```python
from build123d import *

# Parameters (mm, degrees)
SKETCH1_R           = 15
BOSS_EXTRUDE1_DEPTH = 5
SKETCH2_R           = 10
BOSS_EXTRUDE2_DEPTH = 15
SKETCH3_R           = 7.5
CUT_EXTRUDE1_DEPTH  = 19
SKETCH5_R           = 11
BOSS_EXTRUDE3_DEPTH = 1


with BuildPart() as part:
    # Sketch1 → Boss-Extrude1 (new body)
    with BuildSketch(Plane(origin=(0, 0, 0), x_dir=(1, 0, 0), z_dir=(0, 1, 0))):
        Circle(SKETCH1_R)
    extrude(amount=BOSS_EXTRUDE1_DEPTH)

    # Sketch2 → Boss-Extrude2 (add)
    with BuildSketch(Plane(origin=(0, 5, 0), x_dir=(1, 0, 0), z_dir=(0, 1, 0))):
        Circle(SKETCH2_R)
    extrude(amount=BOSS_EXTRUDE2_DEPTH)

    # Sketch3 → Cut-Extrude1 (cut)
    with BuildSketch(Plane.XZ):
        Circle(SKETCH3_R)
    extrude(amount=-CUT_EXTRUDE1_DEPTH, mode=Mode.SUBTRACT)

    # Sketch5 → Boss-Extrude3 (add)
    with BuildSketch(Plane(origin=(0, 5, 0), x_dir=(1, 0, 0), z_dir=(0, 1, 0))):
        Circle(SKETCH5_R)
    extrude(amount=BOSS_EXTRUDE3_DEPTH)


solid = part.part
```
The listing builds one solid part. Answer for the finished solid, in the listing's coordinates (mm). A direction names the side the tool comes from. Give positions to 0.01 mm unless a question says otherwise; leave off trailing zeros. Loops run counter-clockwise (first coordinate to the right, second up) from the corner with the lowest first, then second, coordinate; pieces in that order, holes last. Notation, with made-up numbers: (-12.75, 78) - (5.25, 78) arc R22 ccw to (5.25, 94) - close; hole circle Ø5 at (-10, 63.5). An arc over 180 degrees is marked (long way). Return JSON: item names as keys, results as strings. Group by question number.
1. Straight lines are drawn through the part: line 1 (Y direction, x = 2.5, z = 1.5); line 2 (Z direction, x = 0, y = 12.75); line 3 (Z direction, x = 0, y = 1.8). For each, find the intervals that lie inside material, in ascending order. Write a range as [from, to].
2. Find section A-A (x = 0). Write down the section's boundary in (y, z).
3. Determine the mould class of faces 1 (the cylindrical face through (-14.985, 2.465, -0.66)), 2 (the cylindrical face through (-7.493, 2.465, 0.33)), 3 (the flat face through (0, 6, 0)), 4 (the flat face through (2, 6, 10)) for opening direction Z: pulls with the +Z half, pulls with the -Z half, needs draft (parallel to the pull), parting line crosses it, or undercut.
4. Which of the six approach directions +Z, -Z, +X, -X, +Y, -Y give full straight-line access (tool end or side, diameter ignored) to faces 5 (the flat face through (0, 20, 0)), 6 (the flat face through (0, 5, 0)), 7 (the cylindrical face through (-7.493, 12.409, 0.33)), 8 (the cylindrical face through (-2.17, 12.9, 9.76)), 9 (the flat face through (-4, 0, -7))?
5. Find section D-D (z = -8.25). Write down the section's boundary in (x, y).
6. Find section C-C (y = 4). Write down the section's boundary in (x, z), then the cut area to 3 significant figures.
7. Given pin 1 Ø8 at (y, z) = (16, 0.5) entering from +X; pin 2 Ø1.5 at (x, z) = (-10.5, -10) entering from +Y; pin 3 Ø4 at (y, z) = (5, 11) entering from +X, each flat-ended and moving along its own axis, determine where each tip first touches the part or whether it passes through.
8. Find section B-B (z = 0). Write down the section's boundary in (x, y), then the cut area to 3 significant figures.
Verdict:
{
 "1": {"line 1": "y = [5, 6], [19, 20]", "line 2": "z = [-10, -7.5], [7.5, 10]", "line 3": "z = [-15, -7.5], [7.5, 15]"},
 "2": {"outline": "(0, -15) - (5, -15) - (5, -11) - (6, -11) - (6, -10) - (20, -10) - (20, 10) - (6, 10) - (6, 11) - (5, 11) - (5, 15) - (0, 15) - (0, 7.5) - (5, 7.5) - (5, -7.5) - (0, -7.5) - close; hole (6, -7.5) - (19, -7.5) - (19, 7.5) - (6, 7.5) - close"},
 "3": {"face 1": "parting line crosses it", "face 2": "undercut", "face 3": "undercut", "face 4": "needs draft"},
 "4": {"face 5": "+Z, -Z, +X, -X, +Y", "face 6": "-Y", "face 7": "none", "face 8": "+Y", "face 9": "+Z, -Z, +X, -X, -Y"},
 "5": {"outline": "(-12.53, 0) - (12.53, 0) - (12.53, 5) - (7.28, 5) - (7.28, 6) - (5.65, 6) - (5.65, 20) - (-5.65, 20) - (-5.65, 6) - (-7.28, 6) - (-7.28, 5) - (-12.53, 5) - close"},
 "6": {"outline": "circle Ø30 at (0, 0); hole circle Ø15 at (0, 0)", "area": "530 mm^2"},
 "7": {"pin 1": "stops at x = 10", "pin 2": "stops at y = 5", "pin 3": "stops at x = 12"},
 "8": {"outline": "(-15, 0) - (-7.5, 0) - (-7.5, 5) - (7.5, 5) - (7.5, 0) - (15, 0) - (15, 5) - (11, 5) - (11, 6) - (10, 6) - (10, 20) - (-10, 20) - (-10, 6) - (-11, 6) - (-11, 5) - (-15, 5) - close; hole (-7.5, 6) - (7.5, 6) - (7.5, 19) - (-7.5, 19) - close", "area": "182 mm^2"}
}
